Model file for the job. Use its own axes, mm. A direction names the side the tool comes from. Coordinates: 2 decimals unless noted, no trailing zeros. Write each loop counter-clockwise with the first axis right and the second up, starting at its lowest first coordinate (ties: lowest second). Pieces come first, ordered by that corner, then holes. Notation, with made-up numbers: M 51.5,42.25 L 103.5,42.25 A6 cw 103.5,47.25 Z; hole C -17.5,44.25 d5. An arc over 180 degrees is marked long. Put each result on its own line as item: value. Start each with the question number.
Q1. Which spindle directions (+Z, -Z, +X, -X, +Y, -Y) get a long thin tool onto all of the face, cutting with end or side? Do faces 1 (the cylindrical face through (-15.41, -28.49, 38.61)), 2 (the flat face through (1, 5.656, 25)), 3 (the flat face through (26, 0.246, 20)). Say none if no direction does.
Q2. Cut at D-D (x = 18.5). Write the cut outline in (y, z).
Q3. Drop flat-ended pins along their axis: pin 1 (1.5 mm diameter, centred on x = 9.5, z = 32.5, fed in from -Y); pin 2 (2 mm diameter, centred on y = 2.6, z = 31.6, fed in from -X); pin 3 (10 mm diameter, centred on x = 23, z = 19, fed in from -Y). Give the stop position or say it passes through.
Q4. Drill centre lines: line 1 along Z through (x, y) = (-13, -5); line 2 along Y through (x, z) = (-15, 2); line 3 along X through (y, z) = (-21, 39.5) (3 decimals). Where is each one in solid material? Low to high.
Q5. Pull direction X, two halves, no side cores. Call faces 4 (the cylindrical face through (2.702, 7.983, 15.842)), 5 (the flat face through (-17.875, 1, 20)), 6 (the flat face through (26, -29.574, 38)): pulls with the +X half, pulls with the -X half, needs draft (parallel to the pull), parting line crosses it, or undercut.
Q6. Cut at C-C (z = 31.55). Write the cut outline in (x, y) (3 decimals), then the cut area to 3 significant figures.
Q7. Cut at A-A (z = 38.2). Write the cut outline in (x, y) (3 decimals).
Q8. Cut at B-B (y = -11). Write the cut outline in (x, z) (3 decimals), then the cut area to 3 significant figures.
```python
from build123d import *

# Parameters (mm, degrees)
BOSS_EXTRUDE1_DEPTH = 41
SKETCH2_W           = 5
SKETCH2_H           = 5.6
BOSS_EXTRUDE2_DEPTH = 29.82
FILLET1_R           = 1.5
SKETCH3_R           = 1.35
CUT_EXTRUDE1_DEPTH  = 49
SKETCH4_R           = 1.35
CUT_EXTRUDE2_DEPTH  = 49
SKETCH5_R           = 1.3
SKETCH5_R_2         = 5.25
CUT_EXTRUDE3_DEPTH  = 7


with BuildPart() as part:
    # Sketch1 → Boss-Extrude1 (new body)
    with BuildSketch(Plane.XY):
        Polygon((-17.875, 0.24625), (-12.875, 0.24625), (-12.875, 5.65625), (23.125, 5.65625), (23.125, 0.24625), (28.125, 0.24625), (28.125, 10.24625), (-17.875, 10.24625), align=None)
    extrude(amount=BOSS_EXTRUDE1_DEPTH)

    # Sketch2 → Boss-Extrude2 (add)
    with BuildSketch(Plane.XZ.offset(-0.24625)):
        with Locations((-15.375, 2.8)):
            Rectangle(SKETCH2_W, SKETCH2_H)
        with Locations((-15.375, 38.2)):
            Rectangle(SKETCH2_W, SKETCH2_H)
        with Locations((25.625, 38.2)):
            Rectangle(SKETCH2_W, SKETCH2_H)
        with Locations((25.625, 2.8)):
            Rectangle(SKETCH2_W, SKETCH2_H)
    extrude(amount=BOSS_EXTRUDE2_DEPTH)

    # Fillet1
    fillet1_edges = [part.edges().sort_by_distance(p)[0] for p in [
        (-15.375, -29.57375, 0),
        (-15.375, -29.57375, 5.6),
        (-15.375, -29.57375, 35.4),
        (-15.375, -29.57375, 41),
        (25.625, -29.57375, 41),
        (25.625, -29.57375, 35.4),
        (25.625, -29.57375, 5.6),
        (25.625, -29.57375, 0),
    ]]
    fillet(fillet1_edges, radius=FILLET1_R)

    # Sketch3 → Cut-Extrude1 (cut)
    with BuildSketch(Plane.ZY.offset(17.875)):
        with Locations(Location((38.2, -27.20375, 0), (0, 0, 270))):
            Circle(SKETCH3_R)
        with Locations(Location((2.8, -27.20375, 0), (0, 0, 270))):
            Circle(SKETCH3_R)
        with Locations(Location((38.2, -5.20375, 0), (0, 0, 270))):
            Circle(SKETCH3_R)
        with Locations(Location((2.8, -5.20375, 0), (0, 0, 270))):
            Circle(SKETCH3_R)
    extrude(amount=-CUT_EXTRUDE1_DEPTH, mode=Mode.SUBTRACT)

    # Sketch4 → Cut-Extrude2 (cut)
    with BuildSketch(Plane(origin=(28.125, 0, 0), x_dir=(0, 0, -1), z_dir=(1, 0, 0))):
        with Locations((-9.6, 2.59625)):
            Circle(SKETCH4_R)
        with Locations((-31.6, 2.59625)):
            Circle(SKETCH4_R)
    extrude(amount=-CUT_EXTRUDE2_DEPTH, mode=Mode.SUBTRACT)

    # Sketch5 → Cut-Extrude3 (cut)
    with BuildSketch(Plane(origin=(0, 10.24625, 0), x_dir=(1, 0, 0), z_dir=(0, 1, 0))):
        with Locations(Location((5.125, -9.45, 0), (0, 0, 180))):
            Circle(SKETCH5_R)
        with Locations(Location((-5.924547539, -20.599995905, 0), (0, 0, 180))):
            Circle(SKETCH5_R)
        with Locations(Location((5.125, -31.55, 0), (0, 0, 180))):
            Circle(SKETCH5_R)
        with Locations(Location((16.174547539, -20.599995905, 0), (0, 0, 180))):
            Circle(SKETCH5_R)
        with Locations(Location((5.125, -20.5, 0), (0, 0, 180))):
            Circle(SKETCH5_R_2)
    extrude(amount=-CUT_EXTRUDE3_DEPTH, mode=Mode.SUBTRACT)


solid = part.part
```
Computed values:
1. face 1: +X, -X
1. face 2: +Z, -Z, -Y
1. face 3: +X, -X, -Y
2. outline: M 5.66,0 L 10.25,0 L 10.25,41 L 5.66,41 Z
3. pin 1: y = 5.66
3. pin 2: through
3. pin 3: y = 0.25
4. line 1: 0 to 1.47, 4.13 to 5.6, 35.4 to 36.87, 39.53 to 41
4. line 2: -29.57 to -28.29, -26.12 to -6.29, -4.12 to 10.25
4. line 3: -17.875 to -12.875, 23.125 to 28.125
5. face 4: undercut
5. face 5: pulls with the -X half
5. face 6: needs draft
6. outline: M -17.875,0.246 L -12.875,0.246 L -12.875,1.247 L -17.875,1.247 Z; M -17.875,3.945 L -12.875,3.945 L -12.875,5.656 L 3.825,5.656 L 3.825,10.246 L -17.875,10.246 Z; M 6.425,5.656 L 23.125,5.656 L 23.125,3.945 L 28.125,3.945 L 28.125,10.246 L 6.425,10.246 Z; M 23.125,0.246 L 28.125,0.246 L 28.125,1.247 L 23.125,1.247 Z
6. area: 226 mm2
7. outline: M -17.875,-29.574 L -12.875,-29.574 L -12.875,-28.554 L -17.875,-28.554 Z; M -17.875,-25.854 L -12.875,-25.854 L -12.875,-6.554 L -17.875,-6.554 Z; M -17.875,-3.854 L -12.875,-3.854 L -12.875,5.656 L 23.125,5.656 L 23.125,-3.854 L 28.125,-3.854 L 28.125,10.246 L -17.875,10.246 Z; M 23.125,-29.574 L 28.125,-29.574 L 28.125,-28.554 L 23.125,-28.554 Z; M 23.125,-25.854 L 28.125,-25.854 L 28.125,-6.554 L 23.125,-6.554 Z
8. outline: M -17.875,0 L -12.875,0 L -12.875,5.6 L -17.875,5.6 Z; M -17.875,35.4 L -12.875,35.4 L -12.875,41 L -17.875,41 Z; M 23.125,0 L 28.125,0 L 28.125,5.6 L 23.125,5.6 Z; M 23.125,35.4 L 28.125,35.4 L 28.125,41 L 23.125,41 Z
8. area: 112 mm2
